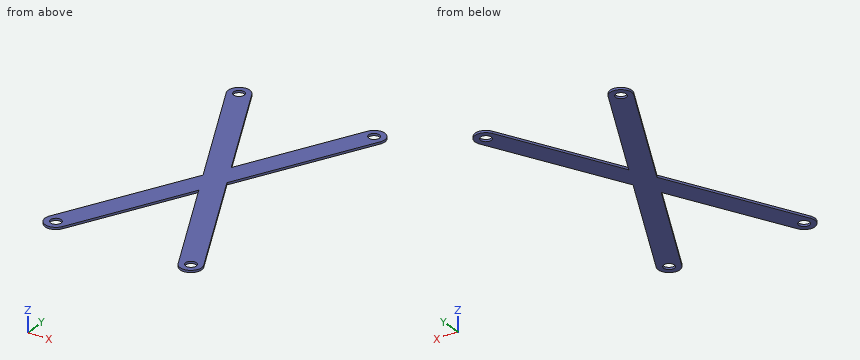
from build123d import *

# Parameters (mm, degrees)
SKETCH_2_R      = 7.5
EXTRUDE_1_DEPTH = 3


with BuildPart() as part:
    # 草图2 → 凸台-拉伸1 (new body)
    with BuildSketch(Plane.XY):
        with BuildLine():
            Line((-13.426802427, 6.687374417), (77.874173312, 190))
            Line((77.874173312, 190), (-13.426802427, 373.312625583))
            ThreePointArc((-13.426802427, 373.312625583), (-6.687374417, 393.426802427), (13.426802427, 386.687374417))
            Line((13.426802427, 386.687374417), (94.6317, 223.645491634))
            Line((94.6317, 223.645491634), (175.836597573, 386.687374417))
            ThreePointArc((175.836597573, 386.687374417), (195.950774417, 393.426802427), (202.690202427, 373.312625583))
            Line((202.690202427, 373.312625583), (111.389226688, 190))
            Line((111.389226688, 190), (202.690202427, 6.687374417))
            ThreePointArc((202.690202427, 6.687374417), (195.950774417, -13.426802427), (175.836597573, -6.687374417))
            Line((175.836597573, -6.687374417), (94.6317, 156.354508366))
            Line((94.6317, 156.354508366), (13.426802427, -6.687374417))
            ThreePointArc((13.426802427, -6.687374417), (-6.687374417, -13.426802427), (-13.426802427, 6.687374417))
        make_face()
        Circle(SKETCH_2_R, mode=Mode.SUBTRACT)
        with Locations((189.2634, 380)):
            Circle(SKETCH_2_R, mode=Mode.SUBTRACT)
        with Locations((189.2634, 0)):
            Circle(SKETCH_2_R, mode=Mode.SUBTRACT)
        with Locations((0, 380)):
            Circle(SKETCH_2_R, mode=Mode.SUBTRACT)
    extrude(amount=EXTRUDE_1_DEPTH)


solid = part.part
Geometry check sheet. Reference: the model listing, model coordinates, mm. Give positions to 0.01 mm unless a question says otherwise; leave off trailing zeros. Order: outer loops, then holes, each group sorted by start corner. A loop starts at its lowest first (then second) coordinate and runs counter-clockwise, first axis right, second up.
1. Depth check by flat-ended pin: pin 1 (1.5 mm diameter, centred on y = 114.5, z = 1.5, fed in from +X); pin 2 (1 mm diameter, centred on x = 111.5, z = 2.5, fed in from -Y); pin 3 (1 mm diameter, centred on x = 106.5, z = 1.5, fed in from +Y). Enter the tip coordinate at first touch or a pass-through.
Completed:
pin 1: stops at x = 149.37
pin 2: stops at y = 121.48
pin 3: stops at y = 248.48
2. Sectioned sample at C-C (y = 0). Record the boundary of the cut face in (x, z).
Completed:
outline: (-15, 0) - (-7.5, 0) - (-7.5, 3) - (-15, 3) - close; (7.5, 0) - (16.76, 0) - (16.76, 3) - (7.5, 3) - close; (172.51, 0) - (181.76, 0) - (181.76, 3) - (172.51, 3) - close; (196.76, 0) - (204.26, 0) - (204.26, 3) - (196.76, 3) - close
3. Scan lines: line 1 (X direction, y = 380, z = 1.75); line 2 (Y direction, x = 0, z = 1.85); line 3 (X direction, y = 120.5, z = 2.15). Record each from-to range of solid material in increasing order.
Completed:
line 1: x = -15 to -7.5, 7.5 to 16.76, 172.51 to 181.76, 196.76 to 204.26
line 2: y = -15 to -7.5, 7.5 to 33.65, 346.35 to 372.5, 387.5 to 395
line 3: x = 43.26 to 76.77, 112.49 to 146
4. Sectioned sample at D-D (x = 0). Record the boundary of the cut face in (y, z), then the cut area to 3 significant figures.
Completed:
outline: (-15, 0) - (-7.5, 0) - (-7.5, 3) - (-15, 3) - close; (7.5, 0) - (33.65, 0) - (33.65, 3) - (7.5, 3) - close; (346.35, 0) - (372.5, 0) - (372.5, 3) - (346.35, 3) - close; (387.5, 0) - (395, 0) - (395, 3) - (387.5, 3) - close
area: 202 mm2
5. Sectioned sample at B-B (y = 271.5). Record the boundary of the cut face in (x, z), then the cut area to 3 significant figures.
Completed:
outline: (37.28, 0) - (70.8, 0) - (70.8, 3) - (37.28, 3) - close; (118.47, 0) - (151.98, 0) - (151.98, 3) - (118.47, 3) - close
area: 201 mm2
6. Sectioned sample at A-A (z = 1.3). Record the boundary of the cut face in (x, y).
Completed:
outline: (-13.43, 6.69) arc R15 ccw to (13.43, -6.69) - (94.63, 156.35) - (175.84, -6.69) arc R15 ccw to (202.69, 6.69) - (111.39, 190) - (202.69, 373.31) arc R15 ccw to (175.84, 386.69) - (94.63, 223.65) - (13.43, 386.69) arc R15 ccw to (-13.43, 373.31) - (77.87, 190) - close; hole circle Ø15 at (0, 0); hole circle Ø15 at (0, 380); hole circle Ø15 at (189.26, 0); hole circle Ø15 at (189.26, 380)
